from build123d import *

# Parameters (mm, degrees)
SKETCH4_W           = 100
SKETCH4_H           = 30
BOSS_EXTRUDE2_DEPTH = 6
CUT_EXTRUDE1_DEPTH  = 105.575331699
SKETCH7_R           = 1.5
CUT_EXTRUDE2_DEPTH  = 105.575331699
FILLET2_R           = 5
FILLET3_R           = 5


with BuildPart() as part:
    # Sketch4 → Boss-Extrude2 (new body)
    with BuildSketch(Plane(origin=(0, 0, 0), x_dir=(1, 0, 0), z_dir=(0, 1, 0))):
        with Locations((50, -15)):
            Rectangle(SKETCH4_W, SKETCH4_H)
    extrude(amount=BOSS_EXTRUDE2_DEPTH)

    # Sketch6 → Cut-Extrude1 (cut, through all)
    with BuildSketch(Plane(origin=(100, 0, 0), x_dir=(0, 0, -1), z_dir=(1, 0, 0))):
        Polygon((-7.5, 0), (0, 0), (0, 4), (-10.856398525, 4), align=None)
        Polygon((-22.5, 0), (-30, 0), (-30, 4), (-19.143601475, 4), align=None)
    extrude(amount=-CUT_EXTRUDE1_DEPTH, mode=Mode.SUBTRACT)

    # Sketch7 → Cut-Extrude2 (cut, through all)
    with BuildSketch(Plane(origin=(0, 6, 0), x_dir=(1, 0, 0), z_dir=(0, 1, 0))):
        with Locations(Location((50, -15, 0), (0, 0, 270))):
            Circle(SKETCH7_R)
    extrude(amount=-CUT_EXTRUDE2_DEPTH, mode=Mode.SUBTRACT)

    # Fillet2
    fillet2_edges = [part.edges().sort_by_distance(p)[0] for p in [
        (0, 5, 0),
    ]]
    fillet(fillet2_edges, radius=FILLET2_R)

    # Fillet3
    fillet3_edges = [part.edges().sort_by_distance(p)[0] for p in [
        (100, 5, 0),
        (100, 5, 30),
        (0, 5, 30),
    ]]
    fillet(fillet3_edges, radius=FILLET3_R)


solid = part.part
CAD build for the part. Positions are in the model's coordinates, mm. A direction names the side the tool comes from. Coordinates: 2 decimals unless noted, no trailing zeros. Loops run counter-clockwise (first coordinate to the right, second up) from the corner with the lowest first, then second, coordinate; pieces in that order, holes last. Notation, with made-up numbers: (29, -11) - (45, -11) arc R9 ccw to (45, 6) - close; hole circle Ø6 at (55.25, 23). An arc over 180 degrees is marked (long way). Write item = value, one per line. Start each with the question number.
Q1. Pull direction X, two halves, no side cores. Call faces 1 (the flat face through (100, 3, 15)), 2 (the flat face through (51, 4, 5)), 3 (the cylindrical face through (48.536, 3.042, 14.675)): pulls with the +X half, pulls with the -X half, needs draft (parallel to the pull), parting line crosses it, or undercut.
Q2. Drill centre lines: L1, parallel to X at y = 1.2, z = 15; L2, parallel to Y at x = 74, z = 26.5; L3, parallel to Y at x = 84, z = 19.5. Where is each one in solid material? Low to high.
Q3. Cut at A-A, the plane x = 50. List the corners of the cut face in (y, z), then the cut area to 3 significant figures.
Q4. Which spindle directions (+Z, -Z, +X, -X, +Y, -Y) get a long thin tool onto all of the face, cutting with end or side? Do faces 4 (the flat face through (51, 4, 25)), 5 (the cylindrical face through (1, 5, 2)). Say none if no direction does.
Q5. Cut at D-D, the plane y = 0.85. List the corners of the cut face in (x, z), then the cut area to 3 significant figures.
Q6. Flat gauge pin, fed straight in: pin 1 Ø2.5 at (x, z) = (50, 15) entering from -Y. Where does the tip first touch, or does it go through?
Q7. Cut at C-C, the plane z = 23.5. List the corners of the cut face in (x, y), then the cut area to 3 significant figures.
Q8. Cut at B-B, the plane z = 15. List the corners of the cut face in (x, y), then the cut area to 3 significant figures.
Computed:
q1.face_1 = pulls with the +X half
q1.face_2 = needs draft
q1.face_3 = undercut
q2.L1 = 0 to 48.5, 51.5 to 100
q2.L2 = 4 to 6
q2.L3 = 0 to 3.58, 4 to 6
q3.outline = (0, 7.5) - (4, 10.86) - (4, 0) - (6, 0) - (6, 13.5) - (0, 13.5) - close; (0, 16.5) - (6, 16.5) - (6, 30) - (4, 30) - (4, 19.14) - (0, 22.5) - close
q3.area = 88.6 mm²
q4.face_4 = +Z, +X, -X
q4.face_5 = -Z, -X, +Y, -Y
q5.outline = (0, 8.21) - (100, 8.21) - (100, 21.79) - (0, 21.79) - close; hole circle Ø3 at (50, 15)
q5.area = 1,350 mm²
q6.pin_1 = through
q7.outline = (0, 4) - (100, 4) - (100, 6) - (0, 6) - close
q7.area = 200 mm²
q8.outline = (0, 0) - (48.5, 0) - (48.5, 6) - (0, 6) - close; (51.5, 0) - (100, 0) - (100, 6) - (51.5, 6) - close
q8.area = 582 mm²
